Verification items for the finished model (mm, model axes). Give positions to 0.01 mm unless a question says otherwise; leave off trailing zeros. Order: outer loops, then holes, each group sorted by start corner. A loop starts at its lowest first (then second) coordinate and runs counter-clockwise, first axis right, second up. Notation, with made-up numbers: (53, 44) -> (103, 44) arc R16 cw to (103, 62) -> close; hole circle Ø9 at (-38.75, 23.5). An arc over 180 degrees is marked (long way). Return JSON: item names as keys, results as strings. Group by question number.
(1) Thickness scan on line 1 along Y through (x, z) = (-19.5, 0.2); line 2 along X through (y, z) = (-20, 0.15); line 3 along X through (y, z) = (48, 1.3). Record the ranges inside material, lowest first.
(2) Cross-section at A-A on z = 1.5. State how many separate pieces and enclosed holes the cut face has, then the cut area to 3 significant figures.
(3) Cross-section at B-B on y = -1. Enter the section's corners in (x, z), then the cut area to 3 significant figures.
(4) Depth check by flat-ended pin: pin 1 Ø2.5 at (x, y) = (15.09, -21.27) entering from -Z. Enter the tip coordinate at first touch or a pass-through.
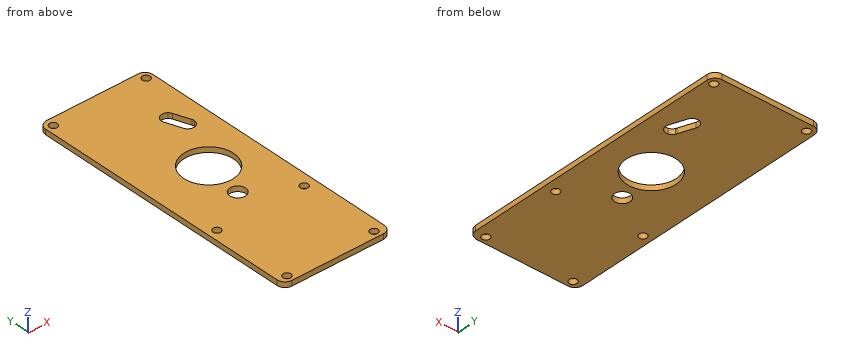
from build123d import *

# Parameters (mm, degrees)
F0_W     = 41
F0_H     = 106
F0_R     = 1.5
F0_R_2   = 5.05
F0_R_3   = 2
F0_R_4   = 3
F0_R_5   = 9.5
F1_DEPTH = 2
F2_R     = 3


# Not quite as in the source:
# - a feature names something its author has since deleted; it is built from what else it names


with BuildPart() as f1:
    # F0 (on Top) → F1 (new body)
    with BuildSketch(Plane.XY):
        with Locations((-1.1801278293, -1.1353523731)):
            Rectangle(F0_W, F0_H)
        with Locations((-18.2301278293, -51.4703523731)):
            Circle(F0_R, mode=Mode.SUBTRACT)
        with Locations((-6.776117335, -33.481924504)):
            Circle(F0_R_2, mode=Mode.SUBTRACT)
        with Locations((-18.2301278293, -21.2703523731)):
            Circle(F0_R, mode=Mode.SUBTRACT)
        with Locations((-11.8353097141, -18.4490393624)):
            Circle(F0_R_3, mode=Mode.SUBTRACT)
        with BuildLine():
            ThreePointArc((0.9913514778, -28.481924504), (-4.9415118708, -25.855220261), (-8.0481067447, -20.1589485871))
            Line((-8.0481067447, -20.1589485871), (9.9913514778, -20.516399593))
            Line((9.9913514778, -20.516399593), (9.9913514778, -46.516399593))
            Line((9.9913514778, -46.516399593), (-8.0481067447, -46.804900421))
            ThreePointArc((-8.0481067447, -46.804900421), (-4.9415118708, -41.1086287471), (0.9913514778, -38.481924504))
            Line((0.9913514778, -38.481924504), (0.9913514778, -28.481924504))
        make_face(mode=Mode.SUBTRACT)
        with Locations((15.0892422113, -51.4703523731)):
            Circle(F0_R, mode=Mode.SUBTRACT)
        with Locations((-1.1801278293, -10.9442314133)):
            Circle(F0_R_4, mode=Mode.SUBTRACT)
        with Locations((15.0892422113, -21.2703523731)):
            Circle(F0_R, mode=Mode.SUBTRACT)
        with Locations((-11.8353097141, -0.1353523731)):
            Circle(F0_R_3, mode=Mode.SUBTRACT)
        with Locations((-11.8353097141, 18.1783346161)):
            Circle(F0_R_3, mode=Mode.SUBTRACT)
        with Locations((-18.8301271707, 48.7366476269)):
            Circle(F0_R, mode=Mode.SUBTRACT)
        with Locations((-6.776117335, 33.2112197578)):
            Circle(F0_R_2, mode=Mode.SUBTRACT)
        with Locations((1.1698721707, 4.2646476269)):
            Circle(F0_R_5, mode=Mode.SUBTRACT)
        with BuildLine():
            ThreePointArc((0.9913514778, 38.2112197578), (-4.9415118708, 40.8379240009), (-8.0481067447, 46.5341956747))
            Line((-8.0481067447, 46.5341956747), (9.9913514778, 46.2456948468))
            Line((9.9913514778, 46.2456948468), (9.9913514778, 31.7237218389))
            ThreePointArc((9.9913514778, 31.7237218389), (10.4081379557, 31.2391097076), (10.6884153726, 30.6646495649))
            Line((10.6884153726, 30.6646495649), (12.8669505005, 24.7255908967))
            ThreePointArc((12.8669505005, 24.7255908967), (12.9813448828, 24.3018570593), (13.0198721707, 23.8646476269))
            ThreePointArc((13.0198721707, 23.8646476269), (12.0896967258, 21.9189727141), (9.9913514778, 21.4211530234))
            Line((9.9913514778, 21.4211530234), (9.9913514778, 20.2456948468))
            Line((9.9913514778, 20.2456948468), (-8.0481067447, 19.8882438409))
            ThreePointArc((-8.0481067447, 19.8882438409), (-4.9415118708, 25.5845155147), (0.9913514778, 28.2112197578))
            Line((0.9913514778, 28.2112197578), (0.9913514778, 38.2112197578))
        make_face(mode=Mode.SUBTRACT)
        with Locations((16.6392421771, 48.7366476269)):
            Circle(F0_R, mode=Mode.SUBTRACT)
        with BuildLine():
            Line((9.9913514778, -20.516399593), (-8.0481067447, -20.1589485871))
            ThreePointArc((-8.0481067447, -20.1589485871), (-4.9415118708, -25.855220261), (0.9913514778, -28.481924504))
            Line((0.9913514778, -28.481924504), (0.9913514778, -38.481924504))
            ThreePointArc((0.9913514778, -38.481924504), (-4.9415118708, -41.1086287471), (-8.0481067447, -46.804900421))
            Line((-8.0481067447, -46.804900421), (9.9913514778, -46.516399593))
            Line((9.9913514778, -46.516399593), (9.9913514778, -20.516399593))
        make_face()
        with Locations((-2.2937730764, -41.981924504)):
            Circle(F0_R, mode=Mode.SUBTRACT)
        with Locations((-2.2937730764, -24.981924504)):
            Circle(F0_R, mode=Mode.SUBTRACT)
        with BuildLine():
            Line((9.9913514778, 46.2456948468), (-8.0481067447, 46.5341956747))
            ThreePointArc((-8.0481067447, 46.5341956747), (-4.9415118708, 40.8379240009), (0.9913514778, 38.2112197578))
            Line((0.9913514778, 38.2112197578), (0.9913514778, 28.2112197578))
            ThreePointArc((0.9913514778, 28.2112197578), (-4.9415118708, 25.5845155147), (-8.0481067447, 19.8882438409))
            Line((-8.0481067447, 19.8882438409), (9.9913514778, 20.2456948468))
            Line((9.9913514778, 20.2456948468), (9.9913514778, 21.4211530234))
            ThreePointArc((9.9913514778, 21.4211530234), (8.9707387909, 21.9024586015), (8.2657292668, 22.7835186943))
            ThreePointArc((8.2657292668, 22.7835186943), (8.1741724057, 22.9999554201), (8.1033430916, 23.2240329142))
            Line((8.1033430916, 23.2240329142), (5.9741724057, 28.9999554201))
            ThreePointArc((5.9741724057, 28.9999554201), (6.9168863609, 31.9338578186), (9.9913514778, 31.7237218389))
            Line((9.9913514778, 31.7237218389), (9.9913514778, 46.2456948468))
        make_face()
        with Locations((-2.2937730764, 24.7112197578)):
            Circle(F0_R, mode=Mode.SUBTRACT)
        with Locations((-2.2937730764, 41.7112197578)):
            Circle(F0_R, mode=Mode.SUBTRACT)
        with Locations((-6.776117335, 33.2112197578)):
            Circle(F0_R_2)
        with Locations((-6.776117335, -33.481924504)):
            Circle(F0_R_2)
        with Locations((-11.8353097141, -18.4490393624)):
            Circle(F0_R_3)
        with Locations((-11.8353097141, -0.1353523731)):
            Circle(F0_R_3)
        with Locations((-11.8353097141, 18.1783346161)):
            Circle(F0_R_3)
        with Locations((-2.2937730764, -24.981924504)):
            Circle(F0_R)
        with Locations((-2.2937730764, -41.981924504)):
            Circle(F0_R)
        with Locations((-2.2937730764, 24.7112197578)):
            Circle(F0_R)
        with Locations((-2.2937730764, 41.7112197578)):
            Circle(F0_R)
    extrude(amount=F1_DEPTH)

    # F2
    f2_edges = [f1.edges().sort_by_distance(p)[0] for p in [
        (-21.680128, 51.864648, 1),
        (-21.680128, -54.135352, 1),
        (19.319872, -54.135352, 1),
        (19.319872, 51.864648, 1),
    ]]
    fillet(f2_edges, radius=F2_R)


solid = f1.part
Verdict:
{
 "1": {"line 1": "-54.02 to -52.27, -50.67 to -22.07, -20.47 to 47.39, 50.08 to 51.75", "line 2": "-21.68 to -19.03, -17.43 to 14.29, 15.89 to 19.32", "line 3": "-21.68 to -20.14, -17.52 to 15.33, 17.95 to 19.32"},
 "2": {"separate pieces": "1", "enclosed holes": "9", "area": "3,930 mm²"},
 "3": {"outline": "(-21.68, 0) -> (-6.74, 0) -> (-6.74, 2) -> (-21.68, 2) -> close; (9.08, 0) -> (19.32, 0) -> (19.32, 2) -> (9.08, 2) -> close", "area": "50.4 mm²"},
 "4": {"pin 1": "through"}
}
